from build123d import *

# Parameters (mm, degrees)
F0_R     = 1.1
F1_DEPTH = 1
F2_W     = 10
F2_H     = 9
F3_DEPTH = 14
F2_W_2   = 14
F4_DEPTH = 11
F6_DEPTH = 25


with BuildPart() as f1:
    # F0 (on Top) → F1 (new body)
    with BuildSketch(Plane.XY):
        with BuildLine():
            ThreePointArc((0, 1), (0.2928932188, 0.2928932188), (1, 0))
            Line((1, 0), (82, 0))
            ThreePointArc((82, 0), (82.7071067812, 0.2928932188), (83, 1))
            Line((83, 1), (83, 49))
            ThreePointArc((83, 49), (82.7071067812, 49.7071067812), (82, 50))
            Line((82, 50), (1, 50))
            ThreePointArc((1, 50), (0.2928932188, 49.7071067812), (0, 49))
            Line((0, 49), (0, 1))
        make_face()
        with Locations((3.5, 3)):
            Circle(F0_R, mode=Mode.SUBTRACT)
        with Locations((79.5, 3)):
            Circle(F0_R, mode=Mode.SUBTRACT)
        with Locations((3.5, 47)):
            Circle(F0_R, mode=Mode.SUBTRACT)
        with Locations((79.5, 47)):
            Circle(F0_R, mode=Mode.SUBTRACT)
    extrude(amount=F1_DEPTH)

    # F2 (on face) → F3 (join)
    with BuildSketch(Plane.XY.offset(1)):
        with Locations((5, 11.5)):
            Rectangle(F2_W, F2_H)
        with Locations((5, 21)):
            Rectangle(F2_W, F2_H)
    extrude(amount=F3_DEPTH)

    # F2 (on face) → F4 (join)
    with BuildSketch(Plane.XY.offset(1)):
        with Locations((7, 34)):
            Rectangle(F2_W_2, F2_H)
    extrude(amount=F4_DEPTH)

    # F5 (on face) → F6 (join)
    with BuildSketch(Plane(origin=(0, 0, 0), x_dir=(0, -1, 0), z_dir=(-1, 0, 0))):
        with BuildLine():
            ThreePointArc((-38.5, 6.5), (-34, 2), (-29.5, 6.5))
            ThreePointArc((-29.5, 6.5), (-34, 11), (-38.5, 6.5))
        make_face()
    extrude(amount=F6_DEPTH)


solid = f1.part
The model under review builds one solid part; all positions refer to its coordinate system, in mm. A direction names the side the tool comes from. Round coordinates to 2 decimals unless told otherwise and drop trailing zeros. Loops run counter-clockwise (first coordinate to the right, second up) from the corner with the lowest first, then second, coordinate; pieces in that order, holes last. Notation, with made-up numbers: M 68,-1.5 L 124,-1.5 A22 cw 124,6.5 Z; hole C 71.5,-30.5 d5. An arc over 180 degrees is marked long. Answer as CSV lines item,"result". Start each with the question number.
Item 1: Insertion check: P1, Ø5, axis at x = 29, z = 2.5, coming from the -Y side; P2, Ø7, axis at x = 7.5, y = 33.5, coming from the +Z side; P3, Ø3, axis at x = 4, z = 7.5, coming from the -Y side; P4, Ø2, axis at y = 14.5, z = 5, coming from the -X side. Each pin has a flat end and moves straight along its axis. Give the tip position at first contact, or say it passes through.
Item 2: For faces 5 (the face through (5, 7, 8)), 6 (the face through (7, 34, 12)), 7 (the face through (78.4, 3, 0.5)), 8 (the face through (5, 16, 8)), 9 (the face through (10, 11, 8)), list the 3-axis set-ups (+Z, -Z, +X, -X, +Y, -Y) from which the entire face can be reached by the end or side of a thin tool; tool diameter is ignored.
Item 3: Consider section C-C (y = 34). Write out the cut boundary in (x, z), then the cut area to 3 significant figures.
Item 4: Consider section D-D (x = 6). Write out the cut boundary in (y, z), then the cut area to 3 significant figures.
Item 5: Wall thickness on line 1 (Y direction, x = 79.5, z = 0.3); line 2 (X direction, y = 23.5, z = 2.25); line 3 (Z direction, x = 46, y = 22.5): over which ranges is each line inside the solid? List them lowest first. Write a range as [from, to].
Item 6: Mouldability with a two-part tool opening along X and no side actions: class faces 1 (the face through (78.4, 47, 0.5)), 2 (the face through (-12.32, 29.84, 4.78)), 3 (the face through (14, 34, 6)), 4 (the face through (0, 20, 6)) as released by +X, released by -X, zero draft, split by the parting line, or undercut.
Item 7: Consider section B-B (z = 10). Write out the cut boundary in (x, y), then the cut area to 3 significant figures.
Item 8: Consider section A-A (x = 79.5). Write out the cut boundary in (y, z), then the cut area to 3 significant figures.
Answer:
1,P1,"stops at y = 0"
1,P2,"stops at z = 12"
1,P3,"stops at y = 7"
1,P4,"stops at x = 0"
2,face 5,"+Z, +X, -X, -Y"
2,face 6,"+Z, +X, -X, +Y"
2,face 7,"+Z, -Z"
2,face 8,"+Z, +X, -X"
2,face 9,"+Z, +X, -Y"
3,outline,"M -25,2 L 0,2 L 0,0 L 83,0 L 83,1 L 14,1 L 14,12 L 0,12 L 0,11 L -25,11 Z"
3,area,"462 mm^2"
4,outline,"M 0,0 L 50,0 L 50,1 L 38.5,1 L 38.5,12 L 29.5,12 L 29.5,1 L 25.5,1 L 25.5,15 L 16.5,15 L 16.5,1 L 16,1 L 16,15 L 7,15 L 7,1 L 0,1 Z"
4,area,"401 mm^2"
5,line 1,"y = [0, 1.9], [4.1, 45.9], [48.1, 50]"
5,line 2,"x = [0, 10]"
5,line 3,"z = [0, 1]"
6,face 1,"undercut"
6,face 2,"zero draft"
6,face 3,"released by +X"
6,face 4,"released by -X"
7,outline,"M -25,31.17 L 0,31.17 L 0,29.5 L 14,29.5 L 14,38.5 L 0,38.5 L 0,36.83 L -25,36.83 Z; M 0,7 L 10,7 L 10,16 L 0,16 Z; M 0,16.5 L 10,16.5 L 10,25.5 L 0,25.5 Z"
7,area,"447 mm^2"
8,outline,"M 0,0 L 1.9,0 L 1.9,1 L 0,1 Z; M 4.1,0 L 45.9,0 L 45.9,1 L 4.1,1 Z; M 48.1,0 L 50,0 L 50,1 L 48.1,1 Z"
8,area,"45.6 mm^2"
